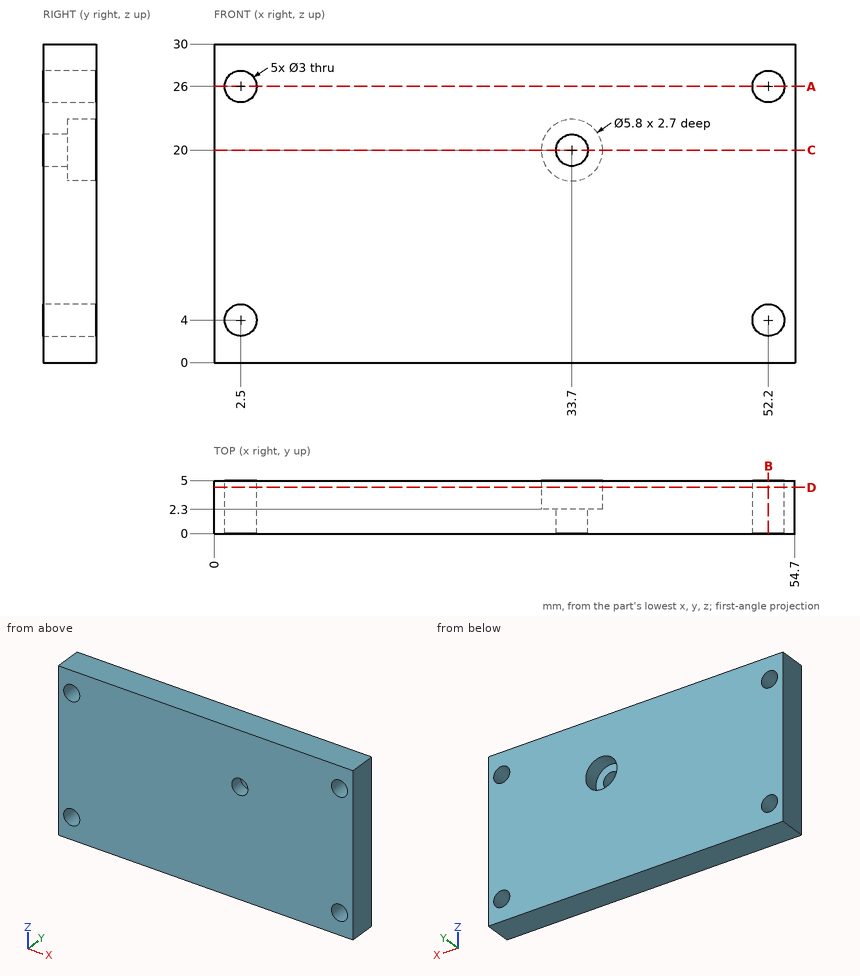
Check sheet for the drawn part. Datum: minimum x, y, z corner. Units: mm. Give positions to 0.01 mm unless a question says otherwise; leave off trailing zeros. Order: outer loops, then holes, each group sorted by start corner. A loop starts at its lowest first (then second) coordinate and runs counter-clockwise, first axis right, second up. Notation, with made-up numbers: (-6.5, 65) - (51.5, 65) arc R28 ccw to (51.5, 86) - close; hole circle Ø2 at (-5.5, -24.5). An arc over 180 degrees is marked (long way). Answer in a Markdown table with one row per item. Add a question column.
Q1. Material ranges on probe 1 along X at (y, z) = (2.7, 26); probe 2 along Z at (x, y) = (33.7, 3.35); probe 3 along Z at (x, y) = (2.5, 1.5), recorded low to high. Write a range as from..to.
Q2. Cross-section at B-B, the plane x = 52.2. Enter the section's corners in (y, z), then the cut area to 3 significant figures.
Q3. Cross-section at C-C, the plane z = 20. Enter the section's corners in (x, y), then the cut area to 3 significant figures.
Q4. Cross-section at A-A, the plane z = 26. Enter the section's corners in (x, y), then the cut area to 4 significant figures.
Q5. Gauge pin test, flat ends, axial feed: pin 1 (1.8 mm diameter, centred on x = 33.7, z = 20, fed in from +Y); pin 2 (1.7 mm diameter, centred on x = 32.5, z = 18.5, fed in from +Y). Record the tip position at first contact, or that the pin passes through.
Q6. Cross-section at D-D, the plane y = 4.35. Enter the section's corners in (x, z), then the cut area to 3 significant figures.
Check values:
| question | item | result |
|---|---|---|
| 1 | probe 1 | x = 0..1, 4..50.7, 53.7..54.7 |
| 1 | probe 2 | z = 0..17.1, 22.9..30 |
| 1 | probe 3 | z = 0..2.5, 5.5..24.5, 27.5..30 |
| 2 | outline | (0, 0) - (5, 0) - (5, 2.5) - (0, 2.5) - close; (0, 5.5) - (5, 5.5) - (5, 24.5) - (0, 24.5) - close; (0, 27.5) - (5, 27.5) - (5, 30) - (0, 30) - close |
| 2 | area | 120 mm^2 |
| 3 | outline | (0, 0) - (32.2, 0) - (32.2, 2.3) - (30.8, 2.3) - (30.8, 5) - (0, 5) - close; (35.2, 0) - (54.7, 0) - (54.7, 5) - (36.6, 5) - (36.6, 2.3) - (35.2, 2.3) - close |
| 3 | area | 251 mm^2 |
| 4 | outline | (0, 0) - (1, 0) - (1, 5) - (0, 5) - close; (4, 0) - (50.7, 0) - (50.7, 5) - (4, 5) - close; (53.7, 0) - (54.7, 0) - (54.7, 5) - (53.7, 5) - close |
| 4 | area | 243.5 mm^2 |
| 5 | pin 1 | passes through |
| 5 | pin 2 | stops at y = 2.3 |
| 6 | outline | (0, 0) - (54.7, 0) - (54.7, 30) - (0, 30) - close; hole circle Ø3 at (2.5, 4); hole circle Ø3 at (2.5, 26); hole circle Ø5.8 at (33.7, 20); hole circle Ø3 at (52.2, 4); hole circle Ø3 at (52.2, 26) |
| 6 | area | 1,590 mm^2 |
